Check sheet for the modelled part. Datum: model origin and axes. Units: mm. Face numbers are marked on the shaded views. A direction names the side the tool comes from. Give positions to 0.01 mm unless a question says otherwise; leave off trailing zeros. Order: outer loops, then holes, each group sorted by start corner. A loop starts at its lowest first (then second) coordinate and runs counter-clockwise, first axis right, second up.
from build123d import *

# Parameters (mm, degrees)
BOSS_EXTRUDE1_DEPTH     = 60
CUT_EXTRUDE4_DEPTH      = 10
CUT_EXTRUDE4_DEPTH_BACK = 10


with BuildPart() as part:
    # Sketch2 → Boss-Extrude1 (new body)
    with BuildSketch(Plane(origin=(0, 0, 0), x_dir=(1, 0, 0), z_dir=(0, 1, 0))):
        with BuildLine():
            Line((-100, 0), (-75, 0))
            ThreePointArc((-75, 0), (0, -75), (75, 0))
            Line((75, 0), (100, 0))
            ThreePointArc((100, 0), (0, -100), (-100, 0))
        make_face()
    extrude(amount=BOSS_EXTRUDE1_DEPTH)

    # Sketch4 → Cut-Extrude4 (cut, two sides)
    with BuildSketch(Plane(origin=(0, 30, 0), x_dir=(1, 0, 0), z_dir=(0, 1, 0))) as cut_extrude4_sk:
        with BuildLine():
            Line((-99.874921777, -5), (-74.833147735, -5))
            ThreePointArc((-74.833147735, -5), (0, -75), (74.833147735, -5))
            Line((74.833147735, -5), (99.874921777, -5))
            ThreePointArc((99.874921777, -5), (0, -100), (-99.874921777, -5))
        make_face()
    extrude(amount=CUT_EXTRUDE4_DEPTH, mode=Mode.SUBTRACT)
    extrude(cut_extrude4_sk.sketch, amount=-CUT_EXTRUDE4_DEPTH_BACK, mode=Mode.SUBTRACT)


solid = part.part
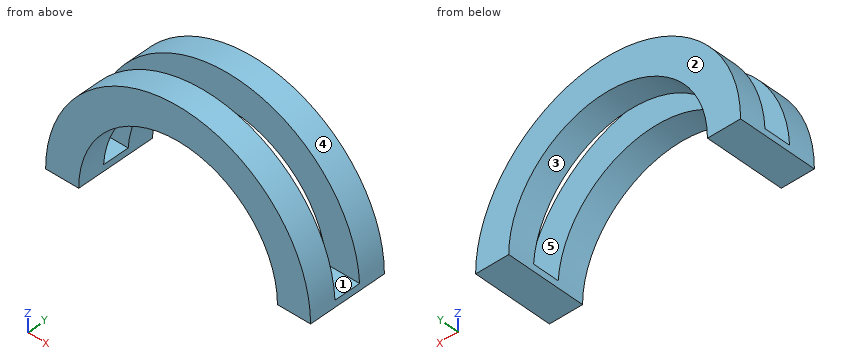
1) Set-up check for the marked faces 1 and 2: record each of +Z, -Z, +X, -X, +Y, -Y from which the full face is reachable in a straight line by a thin tool's end or side.
Recorded:
face 1: +Z, +X, -X
face 2: +Z, -Z, +X, -X, +Y
2) Depth check by flat-ended pin: pin 1 Ø4 at (y, z) = (48.5, 13) entering from -X; pin 2 Ø6 at (y, z) = (47, 82) entering from +X; pin 3 Ø5 at (y, z) = (7, 24) entering from -X. Enter the tip coordinate at first touch or a pass-through.
Recorded:
pin 1: stops at x = -99.39
pin 2: stops at x = 61.31
pin 3: stops at x = -97.66
3) Section check C-C, the plane z = 93. Record the cut outline in (x, y).
Recorded:
outline: (-36.76, 0) - (36.76, 0) - (36.76, 20) - (-36.76, 20) - close; (-36.76, 40) - (36.76, 40) - (36.76, 60) - (-36.76, 60) - close
4) Draft check along X on the marked faces 3, 4 and 5. Enter one of: +X half, -X half, draft (parallel to the pull), parting line (faces both ways), or undercut.
Recorded:
face 3: undercut
face 4: parting line
face 5: draft
5) Section check A-A, the plane x = 0. Record the cut outline in (y, z), then the cut area to 3 significant figures.
Recorded:
outline: (0, 75) - (20, 75) - (20, 100) - (0, 100) - close; (40, 75) - (60, 75) - (60, 100) - (40, 100) - close
area: 1,000 mm2
6) Section check B-B, the plane z = 50. Record the cut outline in (x, y).
Recorded:
outline: (-86.6, 0) - (-55.9, 0) - (-55.9, 20) - (-86.6, 20) - close; (-86.6, 40) - (-55.9, 40) - (-55.9, 60) - (-86.6, 60) - close; (55.9, 0) - (86.6, 0) - (86.6, 20) - (55.9, 20) - close; (55.9, 40) - (86.6, 40) - (86.6, 60) - (55.9, 60) - close
7) Material ranges on L1, parallel to Y at x = 17, z = 81; L2, parallel to Z at x = -78, y = 24; L3, parallel to X at y = 7.5, z = 54, recorded low to high.
Recorded:
L1: y = 0 to 20, 40 to 60
L2: z = 0 to 5
L3: x = -84.17 to -52.05, 52.05 to 84.17
8) Section check D-D, the plane y = 13. Record the cut outline in (x, z), then the cut area to 3 significant figures.
Recorded:
outline: (-100, 0) - (-75, 0) arc R75 cw to (75, 0) - (100, 0) arc R100 ccw to start
area: 6,870 mm2
